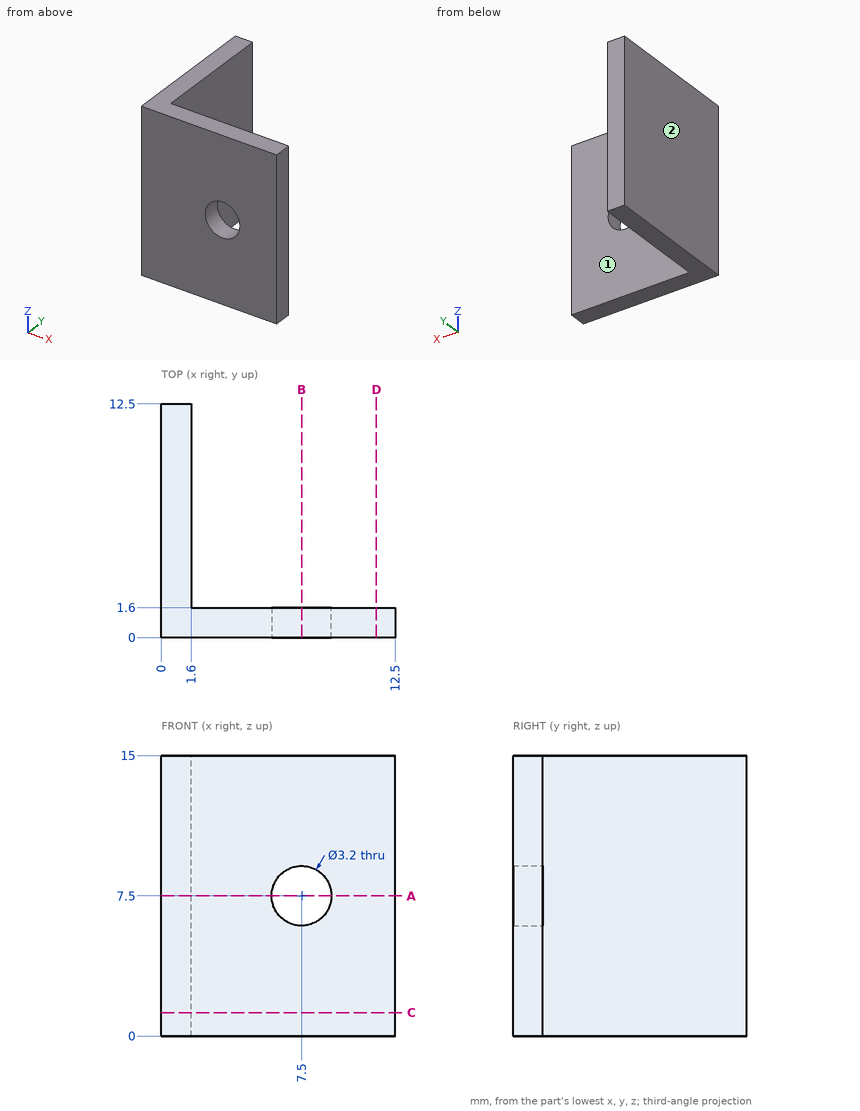
Verification items for this drawing (mm, ordinates from the low corner). A direction names the side the tool comes from. Coordinates: 2 decimals unless noted, no trailing zeros. Write each loop counter-clockwise with the first axis right and the second up, starting at its lowest first coordinate (ties: lowest second). Pieces come first, ordered by that corner, then holes. Notation, with made-up numbers: M 19,-27 L 76,-27 A15 cw 76,-5 Z; hole C -24.5,89.25 d1. An arc over 180 degrees is marked long. Use CSV: the item, a comma, the result in double quotes.
Q1. Go/stop test with flat-tipped pins: P1, Ø3.5, axis at x = 7.5, z = 7.5, coming from the +Y side; P2, Ø4, axis at y = 4.5, z = 10, coming from the +X side. Record where each tip stops, or that it passes through.
Computed values:
P1,"y = 1.6"
P2,"x = 1.6"
Q2. Set-up check for the marked faces 1 and 2: record each of +Z, -Z, +X, -X, +Y, -Y from which the full face is reachable in a straight line by a thin tool's end or side.
Computed values:
face 1,"+Z, -Z, +X, +Y"
face 2,"+Z, -Z, -X, +Y, -Y"
Q3. Thickness scan on line 1 along Z through (x, y) = (7.5, 1); line 2 along Y through (x, z) = (3, 7.75). Record the ranges inside material, lowest first. Write a range as [from, to].
Computed values:
line 1,"[0, 5.9], [9.1, 15]"
line 2,"[0, 1.6]"
Q4. Section check D-D, the plane x = 11.5. Enter the section's corners in (y, z), and give its area (3 significant figures).
Computed values:
outline,"M 0,0 L 1.6,0 L 1.6,15 L 0,15 Z"
area,"24.0 mm²"
Q5. Section check C-C, the plane z = 1.25. Enter the section's corners in (x, y), and give its area (3 significant figures).
Computed values:
outline,"M 0,0 L 12.5,0 L 12.5,1.6 L 1.6,1.6 L 1.6,12.5 L 0,12.5 Z"
area,"37.4 mm²"
Q6. Section check B-B, the plane x = 7.5. Enter the section's corners in (y, z).
Computed values:
outline,"M 0,0 L 1.6,0 L 1.6,5.9 L 0,5.9 Z; M 0,9.1 L 1.6,9.1 L 1.6,15 L 0,15 Z"
Q7. Section check A-A, the plane z = 7.5. Enter the section's corners in (x, y), and give its area (3 significant figures).
Computed values:
outline,"M 0,0 L 5.9,0 L 5.9,1.6 L 1.6,1.6 L 1.6,12.5 L 0,12.5 Z; M 9.1,0 L 12.5,0 L 12.5,1.6 L 9.1,1.6 Z"
area,"32.3 mm²"
